Geometry check sheet. Reference: the model listing, model coordinates, mm. A direction names the side the tool comes from. Round coordinates to 2 decimals unless told otherwise and drop trailing zeros. Loops run counter-clockwise (first coordinate to the right, second up) from the corner with the lowest first, then second, coordinate; pieces in that order, holes last.
```python
from build123d import *

# Parameters (mm, degrees)
F1_DEPTH = 695
F2_W     = 595
F2_H     = 900
F3_DEPTH = 1.2
F4_W     = 509
F4_H     = 299
F5_DEPTH = 10
F4_W_2   = 465
F4_H_2   = 431
F4_W_3   = 10
F6_DEPTH = 10
F7_W     = 465
F7_H     = 605
F7_W_2   = 10
F8_DEPTH = 10
F9_T     = -1.2


# Not quite as in the source:
# - a shell that OpenCascade refuses in one call is made with other operations: the cavity is built on its own and cut out


with BuildPart() as f1:
    # F0 (on Right) → F1 (new body)
    with BuildSketch(Plane.YZ):
        with BuildLine():
            Line((0, 2000), (0, 0))
            Line((0, 0), (865, 0))
            Line((865, 0), (865, 675))
            Line((865, 675), (1265, 675))
            ThreePointArc((1265, 675), (1305, 715), (1265, 755))
            Line((1265, 755), (755.5500969465, 755))
            Line((755.5500969465, 755), (600, 1140))
            Line((600, 1140), (600, 2000))
            Line((600, 2000), (0, 2000))
        make_face()
    extrude(amount=-F1_DEPTH)

    # F2 (on face) → F3 (cut)
    with BuildSketch(Plane.XZ):
        with Locations((-347.5, 1500)):
            Rectangle(F2_W, F2_H)
        with Locations((-347.5, 500)):
            Rectangle(F2_W, F2_H)
    extrude(amount=-F3_DEPTH, mode=Mode.SUBTRACT)

    # F4 (on face) → F5 (cut)
    with BuildSketch(Plane(origin=(0, 600, 0), x_dir=(-1, 0, 0), z_dir=(0, 1, 0))):
        with Locations((347.5, 1329.5)):
            Rectangle(F4_W, F4_H)
    extrude(amount=-F5_DEPTH, mode=Mode.SUBTRACT)

    # F4 (on face) → F6 (cut)
    with BuildSketch(Plane(origin=(0, 600, 0), x_dir=(-1, 0, 0), z_dir=(0, 1, 0))):
        with Locations((347.5, 1719.5)):
            Rectangle(F4_W_2, F4_H_2)
        with Locations((110, 1719.5)):
            Rectangle(F4_W_3, F4_H_2)
        with Locations((585, 1719.5)):
            Rectangle(F4_W_3, F4_H_2)
    extrude(amount=-F6_DEPTH, mode=Mode.SUBTRACT)

    # F7 (on face) → F8 (cut)
    with BuildSketch(Plane(origin=(0, 865, 0), x_dir=(-1, 0, 0), z_dir=(0, 1, 0))):
        with Locations((347.5, 352.5)):
            Rectangle(F7_W, F7_H)
        with Locations((110, 352.5)):
            Rectangle(F7_W_2, F7_H)
        with Locations((585, 352.5)):
            Rectangle(F7_W_2, F7_H)
    extrude(amount=-F8_DEPTH, mode=Mode.SUBTRACT)

    # F9: a shell. OpenCascade refuses it in one call, so the cavity is built on its own and cut out:
    # the body offset inwards by the wall thickness, plus a prism from it out through each open face.
    f9_core = offset(f1.part, amount=F9_T, kind=Kind.INTERSECTION, mode=Mode.PRIVATE)
    f9_exits = [f9_core.faces().sort_by_distance(p)[0] for p in [
        (-347.5, 588.8, 1719.5),
        (-347.5, 588.8, 1329.5),
        (-347.5, 853.8, 352.5),
        (-347.5, 2.4, 500),
        (-347.5, 2.4, 1500),
    ]]
    add(f9_core, mode=Mode.SUBTRACT)
    extrude(f9_exits, amount=-F9_T, mode=Mode.SUBTRACT)


solid = f1.part
```
1) Sectioned sample at A-A, the plane z = 1250. Record the cut outline in (x, y).
Report:
outline: (-695, 0) - (-645, 0) - (-645, 1.2) - (-693.8, 1.2) - (-693.8, 598.8) - (-603.2, 598.8) - (-603.2, 590) - (-602, 590) - (-602, 600) - (-695, 600) - close; (-93, 590) - (-91.8, 590) - (-91.8, 598.8) - (-1.2, 598.8) - (-1.2, 1.2) - (-50, 1.2) - (-50, 0) - (0, 0) - (0, 600) - (-93, 600) - close
2) Sectioned sample at C-C, the plane z = 715. Record the cut outline in (x, y).
Report:
outline: (-695, 0) - (-645, 0) - (-645, 1.2) - (-693.8, 1.2) - (-693.8, 1303.8) - (-1.2, 1303.8) - (-1.2, 1.2) - (-50, 1.2) - (-50, 0) - (0, 0) - (0, 1305) - (-695, 1305) - close
3) Scan lines: line 1 along Z through (x, y) = (-35, 66); line 2 along X through (y, z) = (559.5, 525); line 3 along Z through (x, y) = (-100, 969). Record each from-to range of solid material in increasing order.
Report:
line 1: z = 0 to 1.2, 1998.8 to 2000
line 2: x = -695 to -693.8, -1.2 to 0
line 3: z = 675 to 676.2, 753.8 to 755
4) Access from +Z, -Z, +X, -X, +Y, -Y to the whole of each face (thin tool, end or side, straight path). Record for faces 5 (the face through (-603, 865, 311)), 6 (the face through (-343, 426, 1.2)), 7 (the face through (-603, 600, 1600)), 8 (the face through (-346, 0, 1005)), 9 (the face through (-343, 426, 0)).
Report:
face 5: -Z, +X, -X, +Y
face 6: none
face 7: +Z, +X, -X, +Y
face 8: +Z, -Z, +X, -X, -Y
face 9: -Z, +X, -X, +Y, -Y
5) Sectioned sample at D-D, the plane y = 777. Record the cut outline in (x, z).
Report:
outline: (-695, 0) - (0, 0) - (0, 755) - (-695, 755) - close; hole (-693.8, 1.2) - (-1.2, 1.2) - (-1.2, 753.8) - (-693.8, 753.8) - close
6) Sectioned sample at B-B, the plane y = 382. Record the cut outline in (x, z).
Report:
outline: (-695, 0) - (0, 0) - (0, 2000) - (-695, 2000) - close; hole (-693.8, 1.2) - (-1.2, 1.2) - (-1.2, 1998.8) - (-693.8, 1998.8) - close
7) Gauge pin test, flat end, axial feed: pin 1 (12 mm diameter, centred on x = -224.5, y = 1077, fed in from -Z). Record the tip position at first contact, or that the pin passes through.
Report:
pin 1: stops at z = 675
8) Mould release check, pull along Z, two halves, no side actions. Record for faces 1 (the face through (-349, 1.2, 1005)), 2 (the face through (-695, 353, 1014)), 3 (the face through (-343, 1013, 753.8)), 4 (the face through (-343, 1062, 675)): +Z half, -Z half, draft (parallel to the pull), parting line (faces both ways), or undercut.
Report:
face 1: undercut
face 2: draft
face 3: undercut
face 4: -Z half
